from build123d import *

# Parameters (mm, degrees)
ESBO_O1_W                = 160
ESBO_O1_H                = 20
RESSALTO_EXTRUS_O1_DEPTH = 3
FILETE2_R                = 3


with BuildPart() as part:
    # Esboço1 → Ressalto-extrusão1 (new body)
    with BuildSketch(Plane(origin=(0, 0, 0), x_dir=(1, 0, 0), z_dir=(0, 1, 0))):
        with Locations((41.735785703, -3.037439614)):
            Rectangle(ESBO_O1_W, ESBO_O1_H)
    extrude(amount=RESSALTO_EXTRUS_O1_DEPTH)

    # Filete2
    filete2_edges = [part.edges().sort_by_distance(p)[0] for p in [
        (41.735785703, 3, 13.037439614),
    ]]
    fillet(filete2_edges, radius=FILETE2_R - 0.0001)  # a hair under: the kernel refuses the full size


solid = part.part
CAD build for the part. Positions are in the model's coordinates, mm. Round coordinates to 2 decimals unless told otherwise and drop trailing zeros. Order: outer loops, then holes, each group sorted by start corner. A loop starts at its lowest first (then second) coordinate and runs counter-clockwise, first axis right, second up. Notation, with made-up numbers: (-5.5, 52) -> (37.5, 52) arc R23 cw to (37.5, 66) -> close; hole circle Ø1 at (-29.75, 70.25). An arc over 180 degrees is marked (long way). Write each question's results on one line, items separated by ' | '.
1. Flat gauge pin, fed straight in: P1, Ø1, axis at x = 83, y = 1.5, coming from the +Z side. Where does the tip first touch, or does it go through?
Findings below:
P1: stops at z = 12.87
2. Cut at B-B (y = 2.15). Give the cut face in (x, z).
Findings below:
outline: (-38.26, -6.96) -> (121.74, -6.96) -> (121.74, 12.13) -> (-38.26, 12.13) -> close
3. Wall check: line 1 along Z through (x, y) = (23, 0.3); line 2 along Z through (x, y) = (61.5, 1.95); line 3 along Y through (x, z) = (19, 12). Give the ranges that are in metal, low to high. Write a range as [from, to].
Findings below:
line 1: z = [-6.96, 13.02] | line 2: z = [-6.96, 12.32] | line 3: y = [0, 2.27]
